from build123d import *

# Parameters (mm, degrees)
BOSS_EXTRUDE1_DEPTH = 1.5
SKETCH2_W           = 7
SKETCH2_H           = 2
SKETCH2_W_2         = 2
SKETCH2_H_2         = 7
BOSS_EXTRUDE2_DEPTH = 3
SKETCH3_W           = 23
SKETCH3_H           = 0.5
CUT_EXTRUDE1_DEPTH  = 10
SKETCH4_W           = 23
SKETCH4_H           = 0.5
CUT_EXTRUDE2_DEPTH  = 10
SKETCH5_W           = 0.25
SKETCH5_H           = 4.5
SKETCH5_W_2         = 4
SKETCH5_H_2         = 0.25
CUT_EXTRUDE3_DEPTH  = 10
SKETCH6_W           = 0.5
SKETCH6_H           = 80
SKETCH6_H_2         = 36.75
CUT_EXTRUDE4_DEPTH  = 10


with BuildPart() as part:
    # Sketch1 → Boss-Extrude1 (new body)
    with BuildSketch(Plane(origin=(0, 0, 0), x_dir=(1, 0, 0), z_dir=(0, 1, 0))):
        Polygon((30, 81), (53, 81), (53, 44), (55, 44), (55, 37), (53, 37), (53, 0), (30, 0), (30, -2), (23, -2), (23, 0), (0, 0), (0, 81), (23, 81), (23, 83), (30, 83), align=None)
    extrude(amount=BOSS_EXTRUDE1_DEPTH)

    # Sketch2 → Boss-Extrude2 (add)
    with BuildSketch(Plane(origin=(0, 1.5, 0), x_dir=(1, 0, 0), z_dir=(0, 1, 0))):
        with Locations((26.5, 84)):
            Rectangle(SKETCH2_W, SKETCH2_H)
        with Locations((56, 40.5)):
            Rectangle(SKETCH2_W_2, SKETCH2_H_2)
        with Locations((26.5, -3)):
            Rectangle(SKETCH2_W, SKETCH2_H)
    extrude(amount=-BOSS_EXTRUDE2_DEPTH)

    # Sketch3 → Cut-Extrude1 (cut)
    with BuildSketch(Plane(origin=(0, 1.5, 0), x_dir=(1, 0, 0), z_dir=(0, 1, 0))):
        with Locations((11.5, 80.75)):
            Rectangle(SKETCH3_W, SKETCH3_H)
        with Locations((41.5, 80.75)):
            Rectangle(SKETCH3_W, SKETCH3_H)
    extrude(amount=-CUT_EXTRUDE1_DEPTH, mode=Mode.SUBTRACT)

    # Sketch4 → Cut-Extrude2 (cut)
    with BuildSketch(Plane(origin=(0, 1.5, 0), x_dir=(1, 0, 0), z_dir=(0, 1, 0))):
        with Locations((11.5, 0.25)):
            Rectangle(SKETCH4_W, SKETCH4_H)
        with Locations((41.5, 0.25)):
            Rectangle(SKETCH4_W, SKETCH4_H)
    extrude(amount=-CUT_EXTRUDE2_DEPTH, mode=Mode.SUBTRACT)

    # Sketch5 → Cut-Extrude3 (cut)
    with BuildSketch(Plane(origin=(0, 1.5, 0), x_dir=(1, 0, 0), z_dir=(0, 1, 0))):
        with Locations((23.125, 82.75)):
            Rectangle(SKETCH5_W, SKETCH5_H)
        with Locations((29.875, 82.75)):
            Rectangle(SKETCH5_W, SKETCH5_H)
        with Locations((55, 43.875)):
            Rectangle(SKETCH5_W_2, SKETCH5_H_2)
        with Locations((55, 37.125)):
            Rectangle(SKETCH5_W_2, SKETCH5_H_2)
        with Locations((23.125, -1.75)):
            Rectangle(SKETCH5_W, SKETCH5_H)
        with Locations((29.875, -1.75)):
            Rectangle(SKETCH5_W, SKETCH5_H)
    extrude(amount=-CUT_EXTRUDE3_DEPTH, mode=Mode.SUBTRACT)

    # Sketch6 → Cut-Extrude4 (cut)
    with BuildSketch(Plane(origin=(0, 1.5, 0), x_dir=(1, 0, 0), z_dir=(0, 1, 0))):
        with Locations((0.25, 40.5)):
            Rectangle(SKETCH6_W, SKETCH6_H)
        with Locations((52.75, 18.875)):
            Rectangle(SKETCH6_W, SKETCH6_H_2)
        with Locations((52.75, 62.125)):
            Rectangle(SKETCH6_W, SKETCH6_H_2)
    extrude(amount=-CUT_EXTRUDE4_DEPTH, mode=Mode.SUBTRACT)


solid = part.part
Build history of the part. All positions in model axes, mm. A direction names the side the tool comes from. Coordinates: 2 decimals unless noted, no trailing zeros. Write each loop counter-clockwise with the first axis right and the second up, starting at its lowest first coordinate (ties: lowest second). Pieces come first, ordered by that corner, then holes.
(1) 3-axis set-ups, long thin cutter, end or side, ignore diameter. For faces 1 (the flat face through (55.2, 0.4, -43.75)), 2 (the flat face through (23.25, 0.4, 2.3)), 3 (the flat face through (23.25, 0.4, -83.2)), 4 (the flat face through (29.75, 0.4, 2.3)), 5 (the flat face through (26, -1.5, 3)): which of +Z, -Z, +X, -X, +Y, -Y reach the whole face in a straight line?
(2) Drill centre lines: line 1 (X direction, y = 0.7, z = -73.5); line 2 (Y direction, x = 49, z = -70); line 3 (Z direction, x = 51.5, y = 0.6). Where is each one in solid material? Low to high.
(3) Cut at D-D on x = 32.5. List the corners of the cut face in (y, z).
(4) Cut at A-A on y = -0.9. List the corners of the cut face in (x, z).
(5) Pin check, flat tips, straight feed: pin 1 Ø0.8 at (x, y) = (8, 0.5) entering from +Z; pin 2 Ø0.8 at (y, z) = (0.5, -57.5) entering from +X; pin 3 Ø8 at (x, z) = (19, -65.5) entering from -Y; pin 4 Ø1 at (y, z) = (-1, -58) entering from -X. Stop position of each tip, or through.
(6) Cut at C-C on z = -5. List the corners of the cut face in (x, y), and give its area (3 significant figures).
(7) Cut at B-B on x = 26. List the corners of the cut face in (y, z).
Working result:
1. face 1: -Z, +X, +Y, -Y
1. face 2: +Z, -X, +Y, -Y
1. face 3: -Z, -X, +Y, -Y
1. face 4: +Z, +X, +Y, -Y
1. face 5: +Z, -Z, +X, -X, -Y
2. line 1: x = 0.5 to 52.5
2. line 2: y = 0 to 1.5
2. line 3: z = -80.5 to -0.5
3. outline: (0, -80.5) - (1.5, -80.5) - (1.5, -0.5) - (0, -0.5) - close
4. outline: (23.25, -85) - (29.75, -85) - (29.75, -83) - (23.25, -83) - close; (23.25, 2) - (29.75, 2) - (29.75, 4) - (23.25, 4) - close; (55, -43.75) - (57, -43.75) - (57, -37.25) - (55, -37.25) - close
5. pin 1: stops at z = -0.5
5. pin 2: stops at x = 52.5
5. pin 3: stops at y = 0
5. pin 4: passes through
6. outline: (0.5, 0) - (52.5, 0) - (52.5, 1.5) - (0.5, 1.5) - close
6. area: 78.0 mm2
7. outline: (-1.5, -85) - (1.5, -85) - (1.5, 4) - (-1.5, 4) - (-1.5, 2) - (0, 2) - (0, -83) - (-1.5, -83) - close
